Autodesk Inventor part; units mm, degrees
ref_plane "YZ Plane" through (0, 0, 0) normal (1, 0, 0) x (0, 1, 0)
ref_plane "XZ Plane" through (0, 0, 0) normal (0, 1, 0) x (-1, 0, 0)
ref_plane "XY Plane" through (0, 0, 0) normal (0, 0, 1) x (1, 0, 0)
sketch "Sketch1" plane through (0, 0, 0) normal (0, 0, 1) x (1, 0, 0)
  line L0 (0, 0) -> (127, 0)
  line L1 (127, 0) -> (127, 177.8)
  line L2 (127, 177.8) -> (0, 177.8)
  line L3 (0, 177.8) -> (0, 0)
  dimension "d0" = 127
  dimension "d1" = 177.8
extrude "Extrusion1" add sketch "Sketch1" against normal blind 12.7
sketch "Sketch2" plane through (0, 0, 0) normal (0, 0, 1) x (1, 0, 0)
  line L0 (0, 0) -> (0, 177.8)
  line L1 (127, 177.8) -> (127, 0)
  line L2 (25.4, 158.75) -> (101.6, 158.75)
  line L3 (101.6, 158.75) -> (101.6, 165.1)
  line L4 (101.6, 165.1) -> (25.4, 165.1)
  line L5 (25.4, 165.1) -> (25.4, 158.75)
  line L6 (25.4, 19.05) -> (101.6, 19.05)
  line L7 (101.6, 19.05) -> (101.6, 12.7)
  line L8 (101.6, 12.7) -> (25.4, 12.7)
  line L9 (25.4, 12.7) -> (25.4, 19.05)
  point P0 (63.5, 158.75)
  point P1 (101.6, 158.75)
  point P2 (63.5, 41.3327)
  dimension "d25" = 6.35
  dimension "d26" = 6.35
sketch "Sketch3" plane through (0, 0, 0) normal (0, 0, 1) x (1, 0, 0)
  point P0 (0, 0)
sketch "Sketch4" plane through (0, 0, 0) normal (0, 0, 1) x (1, 0, 0)
  line L0 (38.1, 63.5) -> (90.6923, 63.5)
  line L1 (90.6923, 63.5) -> (90.6923, 111.7968)
  line L2 (90.6923, 111.7968) -> (38.1, 111.7968)
  line L3 (38.1, 111.7968) -> (38.1, 63.5)
  point P0 (0, 0)
extrude "Extrusion2" add sketch "Sketch4" along normal blind 44.45
sketch "Sketch5" plane through (38.1, 63.5, 0) normal (-1, 0, 0) x (0, 0, 1)
  circle A0 centre (19.05, 37.0546) radius 6.35
  circle A1 centre (33.02, 41.2603) radius 3.175
  circle A2 centre (33.02, 31.5839) radius 3.175
  circle A3 centre (33.02, 23.1169) radius 3.175
  circle A4 centre (33.02, 14.4772) radius 3.175
  circle A5 centre (33.02, 5.8375) radius 3.175
  line L0 (0, 114.3) -> (0, -63.5)
  line L1 (44.45, 48.2968) -> (44.45, 0)
  dimension "d10" = 6.35
  dimension "d29" = 19.05
  dimension "d30" = 11.43
  dimension "d31" = 11.43
  dimension "d32" = 11.43
  dimension "d33" = 11.43
  dimension "d34" = 11.43
extrude "Extrusion3" cut sketch "Sketch5" against normal blind 254 contours A0
extrude "Extrusion5" cut sketch "Sketch5" against normal blind 254 contours A1 | A2 | A3 | A4
sketch "Sketch6" plane through (0, 0, 44.45) normal (0, 0, 1) x (1, 0, 0)
  line L0 (38.1, 107.9353) -> (90.6923, 107.9353)
  line L1 (41.91, 67.31) -> (86.0576, 67.31)
  line L2 (86.0576, 67.31) -> (86.0576, 107.9353)
  line L3 (86.0576, 107.9353) -> (41.91, 107.9353)
  line L4 (41.91, 107.9353) -> (41.91, 67.31)
  point P0 (0, 0)
extrude "Extrusion6" cut sketch "Sketch6" against normal blind 34.29
sketch "Sketch7" plane through (38.1, 111.7968, 0) normal (0, 1, 0) x (1, 0, 0)
  line L0 (3.81, -44.45) -> (3.81, -33.02)
  line L1 (3.81, -10.16) -> (47.9576, -10.16)
  line L2 (3.81, -38.735) -> (47.9576, -38.735)
  line L3 (47.9576, -38.735) -> (47.9576, -10.16)
  line L4 (47.9576, -10.16) -> (3.81, -10.16)
  line L5 (3.81, -10.16) -> (3.81, -38.735)
  line L6 (3.81, -38.735) -> (47.9576, -38.735)
  line L7 (47.9576, -38.735) -> (47.9576, -50.1618)
  line L8 (47.9576, -50.1618) -> (3.81, -50.1618)
  line L9 (3.81, -50.1618) -> (3.81, -38.735)
  point P0 (-38.1, 0)
extrude "Extrusion7" cut sketch "Sketch7" against normal blind 34.29 contours L0 L5 L1 L3 L2
extrude "Extrusion8" cut sketch "Sketch7" against normal blind 34.29 contours L0 L2 L7 L8 L9
extrude "Extrusion11" cut sketch "Sketch2" against normal blind 25.4
sketch "Sketch8" plane through (38.1, 111.7968, 0) normal (0, 1, 0) x (1, 0, 0)
  line L0 (47.9576, -10.16) -> (3.81, -10.16)
  line L1 (63.5, 0) -> (-12.7, 0)
  line L2 (3.81, -10.16) -> (47.9681, -10.16)
  line L3 (47.9681, -10.16) -> (47.9681, 0)
  line L4 (47.9681, 0) -> (3.81, 0)
  line L5 (3.81, 0) -> (3.81, -10.16)
  point P0 (-38.1, 0)
extrude "Extrusion12" cut sketch "Sketch8" against normal blind 44.45
fillet "Fillet1" radius 3.175 6 edges at (0, 177.8, -6.35) (127, 177.8, -6.35) (63.5, 177.8, 0) (127, 88.9, 0) (0, 88.9, 0) (63.5, 0, 0)
properties part number "LucasCharles Part 1 wall mount FINAL v2" material "Stainless Steel, Austenitic"
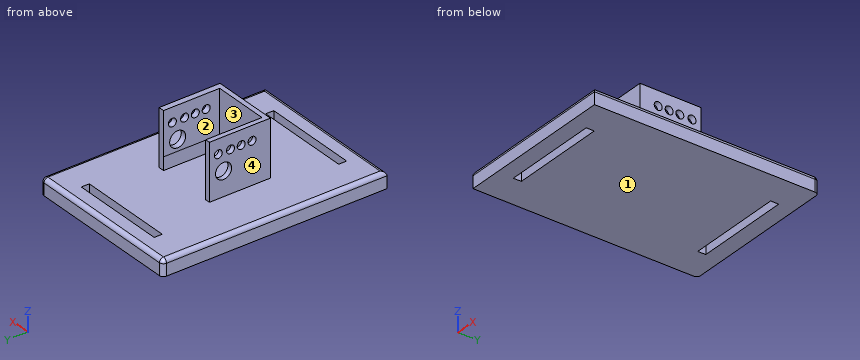
Here's how the part is built. I have some questions about the finished solid (model axes, mm). Face numbers are marked on the shaded views. Coordinates: 2 decimals unless noted, no trailing zeros. Loops run counter-clockwise (first coordinate to the right, second up) from the corner with the lowest first, then second, coordinate; pieces in that order, holes last. Notation, with made-up numbers: M -34.75,-27.5 L 7.25,-27.5 A21 cw 7.25,-13.5 Z; hole C -35.75,-28.75 d7. An arc over 180 degrees is marked long. One line per item, written item: value.
1. Imagine slicing it at B-B (x = 51). List the corners of the cut face in (y, z) for me (3 decimals), and give its area (3 significant figures).
Geometry says:
outline: M 0,-12.7 L 12.7,-12.7 L 12.7,0 L 3.175,0 A3.175 ccw 0,-3.175 Z; M 19.05,-12.7 L 158.75,-12.7 L 158.75,0 L 67.347,0 L 67.347,10.16 L 67.31,10.16 L 67.31,44.45 L 63.5,44.45 L 63.5,0 L 19.05,0 Z; M 165.1,-12.7 L 177.8,-12.7 L 177.8,-3.175 A3.175 ccw 174.625,0 L 165.1,0 Z
area: 2,260 mm2
2. Please list where these lines run through material, in increasing order: probe 1 along Y at (x, z) = (87, 33.02); probe 2 along X at (y, z) = (70, 16); probe 3 along Z at (x, y) = (16, 14.5).
Geometry says:
probe 1: y = 63.5 to 74.8, 81.15 to 83.44, 89.79 to 91.91, 98.26 to 101.59, 107.94 to 111.8
probe 2: x = 38.1 to 41.91, 86.06 to 90.69
probe 3: z = -12.7 to 0
3. Imagine slicing it at C-C (z = 28). List the corners of the cut face in (x, y) for me, and give its area (3 significant figures).
Geometry says:
outline: M 38.1,63.5 L 90.69,63.5 L 90.69,111.8 L 86.06,111.8 L 86.06,67.31 L 41.91,67.31 L 41.91,111.8 L 38.1,111.8 Z
area: 576 mm2
4. Thinking about a two-plate mould opening in X: for the marked faces 1, 2, 3 and 4, which applies, +X half, -X half, draft (parallel to the pull), parting line (faces both ways), or undercut?
Geometry says:
face 1: draft
face 2: undercut
face 3: undercut
face 4: -X half
5. Will these pins go through, and if not, where does the flat tip stop? pin 1 Ø13.5 at (y, z) = (96.5, 17) entering from +X; pin 2 Ø6 at (x, z) = (84, 33) entering from -Y; pin 3 Ø2.5 at (x, z) = (88, 16.5) entering from +Y.
Geometry says:
pin 1: stops at x = 90.69
pin 2: stops at y = 63.5
pin 3: stops at y = 111.8
6. Imagine slicing it at D-D (z = -6). List the corners of the cut face in (x, y) for me (3 decimals).
Geometry says:
outline: M 0,0 L 127,0 L 127,174.625 A3.175 ccw 123.825,177.8 L 3.175,177.8 A3.175 ccw 0,174.625 Z; hole M 25.4,12.7 L 101.6,12.7 L 101.6,19.05 L 25.4,19.05 Z; hole M 25.4,158.75 L 101.6,158.75 L 101.6,165.1 L 25.4,165.1 Z
7. Imagine slicing it at A-A (z = 19.05). List the corners of the cut face in (x, y) for me.
Geometry says:
outline: M 38.1,63.5 L 90.69,63.5 L 90.69,94.2 L 86.06,94.2 L 86.06,67.31 L 41.91,67.31 L 41.91,94.2 L 38.1,94.2 Z; M 38.1,106.9 L 41.91,106.9 L 41.91,111.8 L 38.1,111.8 Z; M 86.06,106.9 L 90.69,106.9 L 90.69,111.8 L 86.06,111.8 Z
